Geometry check sheet. Reference: the model listing, model coordinates, mm. A direction names the side the tool comes from. Give positions to 0.01 mm unless a question says otherwise; leave off trailing zeros. Write each loop counter-clockwise with the first axis right and the second up, starting at its lowest first coordinate (ties: lowest second). Pieces come first, ordered by that corner, then holes. Notation, with made-up numbers: (5, 89) - (51, 89) arc R18 ccw to (51, 101) - close; hole circle Ø7 at (85, 22). An arc over 180 degrees is marked (long way). Write item = value, one per line. Start each with the question number.
(1) Depth check by flat-ended pin: pin 1 Ø2.5 at (x, z) = (-0.5, 0.5) entering from +Y; pin 2 Ø1.1 at (y, z) = (20, -5.5) entering from -X; pin 3 Ø3 at (x, z) = (5.5, -2) entering from +Y. Enter the tip coordinate at first touch or a pass-through.
(2) Section check B-B, the plane y = 22.5. Enter the section's corners in (x, z), plus the area to 3 significant figures.
(3) Section check A-A, the plane y = 3. Enter the section's corners in (x, z).
(4) Section check C-C, the plane y = 10. Enter the section's corners in (x, z), plus the area to 3 significant figures.
(5) Thickness scan on L1, parallel to Z at x = 0, y = 3; L2, parallel to Y at x = 2.5, z = 5; L3, parallel to Z at x = 0, y = 5. Record the ranges inside material, lowest first.
(6) Access from +Z, -Z, +X, -X, +Y, -Y to the whole of each face (thin tool, end or side, straight path). Record for faces 4 (the cylindrical face through (0, 3, -1)), 5 (the flat face through (0, 21, 0)), 6 (the flat face through (-1.5, 19.3, -5.4)), 7 (the cylindrical face through (5.979, 3.94, -3.387)).
(7) Draft check along Z on faces 1 (the cylindrical face through (-1.19, 9.42, -5.37)), 2 (the flat face through (0, 20, -5.892)), 3 (the cylindrical face through (-1.5, 17.96, -0.07)). Enter one of: pulls with the +Z half, pulls with the -Z half, needs draft (parallel to the pull), parting line crosses it, or undercut.
```python
from build123d import *

# Parameters (mm, degrees)
SKETCH_R      = 5.5
PAD_DEPTH     = 15
SKETCH001_R   = 6
PAD001_DEPTH  = 2
SKETCH002_R   = 1.5
PAD002_DEPTH  = 6
SKETCH003_W   = 3
SKETCH003_H   = 1
PAD003_DEPTH  = 10
SKETCH004_R   = 2.85
SKETCH004_R_2 = 1
POCKET_DEPTH  = 10
FILLET_R      = 1.2
FILLET001_R   = 0.4
SKETCH005_R   = 5
PAD004_DEPTH  = 3
FILLET002_R   = 0.2


with BuildPart() as part:
    # Sketch → Pad (new body)
    with BuildSketch(Plane.XZ):
        Circle(SKETCH_R)
    extrude(amount=-PAD_DEPTH)

    # Sketch001 → Pad001 (join)
    with BuildSketch(Plane.XZ):
        Circle(SKETCH001_R)
    extrude(amount=PAD001_DEPTH)

    # Sketch002 (on Face5 of Pad001) → Pad002 (join)
    with BuildSketch(Plane(origin=(0, 15, 0), x_dir=(1, 0, 0), z_dir=(0, 1, 0))):
        Circle(SKETCH002_R)
    extrude(amount=PAD002_DEPTH)

    # Sketch003 (on Face5 of Pad002) → Pad003 (join)
    with BuildSketch(Plane(origin=(0, 15, 0), x_dir=(1, 0, 0), z_dir=(0, 1, 0))):
        with Locations((0, 5.391628)):
            Rectangle(SKETCH003_W, SKETCH003_H)
    extrude(amount=PAD003_DEPTH)

    # Sketch004 (on Face3 of Pad003) → Pocket (cut)
    with BuildSketch(Plane.XZ.offset(2)):
        Circle(SKETCH004_R)
        Circle(SKETCH004_R_2, mode=Mode.SUBTRACT)
    extrude(amount=-POCKET_DEPTH, mode=Mode.SUBTRACT)

    # Fillet
    fillet_edges = [part.edges().sort_by_distance(p)[0] for p in [
        (1.5, 25, -5.391628),
        (-1.5, 25, -5.391628),
    ]]
    fillet(fillet_edges, radius=FILLET_R)

    # Fillet001
    fillet001_edges = [part.edges().sort_by_distance(p)[0] for p in [
        (-6, -2, 0),
        (-6, 0, 0),
        (-1, -2, 0),
    ]]
    fillet(fillet001_edges, radius=FILLET001_R)

    # Sketch005 (on DatumPlane) → Pad004 (join)
    with BuildSketch(Plane.XZ.offset(-1)):
        Polygon((4, -6.928203), (8, 0), (4, 6.928203), (-4, 6.928203), (-8, 0), (-4, -6.928203), align=None)
        Circle(SKETCH005_R, mode=Mode.SUBTRACT)
    extrude(amount=-PAD004_DEPTH)

    # Fillet002
    fillet002_edges = [part.edges().sort_by_distance(p)[0] for p in [
        (0, 1, -6.928203),
        (6, 1, -3.464102),
        (0, 1, 6.928203),
        (6, 1, 3.464102),
        (-6, 1, -3.464102),
        (-6, 1, 3.464102),
        (-6, 4, 3.464102),
        (-6, 4, -3.464102),
        (0, 4, 6.928203),
        (6, 4, 3.464102),
        (6, 4, -3.464102),
        (0, 4, -6.928203),
    ]]
    fillet(fillet002_edges, radius=FILLET002_R)


solid = part.part
```
Model answer:
q1.pin_1 = 21
q1.pin_2 = -1.5
q1.pin_3 = 15
q2.outline = (-1.5, -5.89) - (1.5, -5.89) - (1.5, -4.89) - (-1.5, -4.89) - close
q2.area = 3.00 mm²
q3.outline = (-8, 0) - (-4, -6.93) - (4, -6.93) - (8, 0) - (4, 6.93) - (-4, 6.93) - close; circle Ø2 at (0, 0); hole circle Ø5.7 at (0, 0)
q4.outline = circle Ø11 at (0, 0)
q4.area = 95.0 mm²
q5.L1 = -6.93 to -2.85, -1 to 1, 2.85 to 6.93
q5.L2 = -2 to 0, 1 to 4
q5.L3 = -5.5 to -2.85, -1 to 1, 2.85 to 5.5
q6.face_4 = -Y
q6.face_5 = +Z, +X, -X, +Y
q6.face_6 = +Z, -Z, -X, +Y
q6.face_7 = -Z, +X, +Y
q7.face_1 = parting line crosses it
q7.face_2 = pulls with the -Z half
q7.face_3 = undercut
